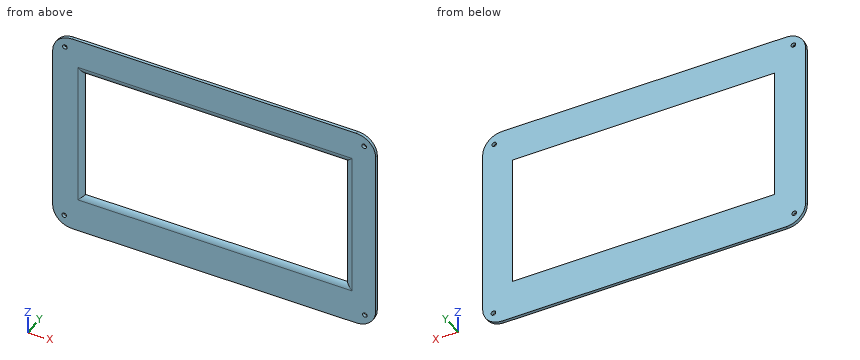
from build123d import *

# Parameters (mm, degrees)
F0_W         = 170.18
F0_H         = 87.63
F1_DEPTH     = 2
F3_D         = 3
F4_T1_DEPTH  = 87.63
F4_T3_DEPTH  = 170.18
F4_T9_DEPTH  = 97.7295049384
F4_T13_DEPTH = 180.2795049384
F4_T20_DEPTH = 97.7295049384
F4_T24_DEPTH = 180.2795049384
F4_T31_DEPTH = 180.2795049384
F4_T35_DEPTH = 97.7295049384
F4_T42_DEPTH = 180.2795049384
F4_T46_DEPTH = 97.7295049384


# Not quite as in the source:
# - a fillet or chamfer that OpenCascade refuses, or shapes differently, is made with other operations: its cross-section is extruded or revolved along the edge and cut away or added


with BuildPart() as f1:
    # F0 (on Front) → F1 (new body)
    with BuildSketch(Plane.XZ):
        with BuildLine():
            Line((94.3139557123, 80.8203592896), (-90.2860442877, 80.8203592896))
            ThreePointArc((-90.2860442877, 80.8203592896), (-99.2663004088, 77.1006154107), (-102.9860442877, 68.1203592896))
            Line((-102.9860442877, 68.1203592896), (-102.9860442877, -43.4872407104))
            ThreePointArc((-102.9860442877, -43.4872407104), (-99.2663004088, -52.4674968314), (-90.2860442877, -56.1872407104))
            Line((-90.2860442877, -56.1872407104), (94.3139557123, -56.1872407104))
            ThreePointArc((94.3139557123, -56.1872407104), (103.2942118334, -52.4674968314), (107.0139557123, -43.4872407104))
            Line((107.0139557123, -43.4872407104), (107.0139557123, 68.1203592896))
            ThreePointArc((107.0139557123, 68.1203592896), (103.2942118334, 77.1006154107), (94.3139557123, 80.8203592896))
        make_face()
        with Locations((2.4907932702, 13.8051814874)):
            Rectangle(F0_W, F0_H, mode=Mode.SUBTRACT)
    extrude(amount=F1_DEPTH)

    # F3 (through all)
    with Locations(Plane.XZ.offset(2)):
        with Locations((-95.5433249474, -48.3972094953), (-95.0444117188, 73.3367204666), (100.0292077661, -48.3972094953), (99.5303019881, 73.3367204666)):
            Hole(F3_D / 2)

    # F4: fillet of radius 5.08 on 4 edges, made by hand

    # F4_s2 → F4_t1 (cut)
    with BuildSketch(Plane.XY.offset(-30.0098185126)):
        with BuildLine():
            ThreePointArc((91.6205952456, -2), (89.3667097117, -1.4726256161), (87.5807932702, 0))
            Line((87.5807932702, 0), (87.5807932702, -2))
            Line((87.5807932702, -2), (91.6205952456, -2))
        make_face()
        with BuildLine():
            ThreePointArc((-86.6390087051, -2), (-84.3851231712, -1.4726256161), (-82.5992067298, 0))
            Line((-82.5992067298, 0), (-82.5992067298, -2))
            Line((-82.5992067298, -2), (-86.6390087051, -2))
        make_face()
    extrude(amount=F4_T1_DEPTH, mode=Mode.SUBTRACT)

    # F4_s4 → F4_t3 (cut)
    with BuildSketch(Plane.YZ.offset(-82.5992067298)):
        with BuildLine():
            ThreePointArc((-2, 61.6599834627), (-1.4726256161, 59.4060979288), (0, 57.6201814874))
            Line((0, 57.6201814874), (-2, 57.6201814874))
            Line((-2, 57.6201814874), (-2, 61.6599834627))
        make_face()
        with BuildLine():
            ThreePointArc((-2, -34.049620488), (-1.4726256161, -31.795734954), (0, -30.0098185126))
            Line((0, -30.0098185126), (-2, -30.0098185126))
            Line((-2, -30.0098185126), (-2, -34.049620488))
        make_face()
    extrude(amount=F4_T3_DEPTH, mode=Mode.SUBTRACT)


with BuildPart() as f4_tool7:
    # F4_s8 → F4_t9 (new body)
    with BuildSketch(Plane.XY.offset(67.7196864257)):
        with BuildLine():
            ThreePointArc((91.6205952456, -2), (89.3667097117, -1.4726256161), (87.5807932702, 0))
            Line((87.5807932702, 0), (87.5807932702, -2))
            Line((87.5807932702, -2), (91.6205952456, -2))
        make_face()
    extrude(amount=-F4_T9_DEPTH)

    split(bisect_by=Plane.XY.offset(57.6201814874), keep=Keep.TOP)


with BuildPart() as f4_tool11:
    # F4_s12 → F4_t13 (new body)
    with BuildSketch(Plane.YZ.offset(-82.5992067298)):
        with BuildLine():
            ThreePointArc((-2, 61.6599834627), (-1.4726256161, 59.4060979288), (0, 57.6201814874))
            Line((0, 57.6201814874), (-2, 57.6201814874))
            Line((-2, 57.6201814874), (-2, 61.6599834627))
        make_face()
    extrude(amount=F4_T13_DEPTH)

    split(bisect_by=Plane.YZ.offset(87.5807932702), keep=Keep.TOP)


with BuildPart() as f4_tool7_1:
    add(f4_tool7.part)

    # F4_t15: intersect F4_tool11
    add(f4_tool11.part, mode=Mode.INTERSECT)


with BuildPart() as f1_1:
    add(f1.part)

    # F4_t5: cut F4_tool7
    add(f4_tool7_1.part, mode=Mode.SUBTRACT)


with BuildPart() as f4_tool18:
    # F4_s19 → F4_t20 (new body)
    with BuildSketch(Plane.XY.offset(57.6201814874)):
        with BuildLine():
            ThreePointArc((91.6205952456, -2), (89.3667097117, -1.4726256161), (87.5807932702, 0))
            Line((87.5807932702, 0), (87.5807932702, -2))
            Line((87.5807932702, -2), (91.6205952456, -2))
        make_face()
    extrude(amount=-F4_T20_DEPTH)

    split(bisect_by=Plane.XY.offset(-30.0098185126), keep=Keep.BOTTOM)


with BuildPart() as f4_tool22:
    # F4_s23 → F4_t24 (new body)
    with BuildSketch(Plane.YZ.offset(97.6802982086)):
        with BuildLine():
            ThreePointArc((-2, -34.049620488), (-1.4726256161, -31.795734954), (0, -30.0098185126))
            Line((0, -30.0098185126), (-2, -30.0098185126))
            Line((-2, -30.0098185126), (-2, -34.049620488))
        make_face()
    extrude(amount=-F4_T24_DEPTH)

    split(bisect_by=Plane.YZ.offset(87.5807932702), keep=Keep.TOP)


with BuildPart() as f4_tool18_1:
    add(f4_tool18.part)

    # F4_t26: intersect F4_tool22
    add(f4_tool22.part, mode=Mode.INTERSECT)


with BuildPart() as f1_2:
    add(f1_1.part)

    # F4_t16: cut F4_tool18
    add(f4_tool18_1.part, mode=Mode.SUBTRACT)


with BuildPart() as f4_tool29:
    # F4_s30 → F4_t31 (new body)
    with BuildSketch(Plane.YZ.offset(-92.6987116681)):
        with BuildLine():
            ThreePointArc((-2, 61.6599834627), (-1.4726256161, 59.4060979288), (0, 57.6201814874))
            Line((0, 57.6201814874), (-2, 57.6201814874))
            Line((-2, 57.6201814874), (-2, 61.6599834627))
        make_face()
    extrude(amount=F4_T31_DEPTH)

    split(bisect_by=Plane.YZ.offset(-82.5992067298), keep=Keep.BOTTOM)


with BuildPart() as f4_tool33:
    # F4_s34 → F4_t35 (new body)
    with BuildSketch(Plane.XY.offset(-30.0098185126)):
        with BuildLine():
            ThreePointArc((-86.6390087051, -2), (-84.3851231712, -1.4726256161), (-82.5992067298, 0))
            Line((-82.5992067298, 0), (-82.5992067298, -2))
            Line((-82.5992067298, -2), (-86.6390087051, -2))
        make_face()
    extrude(amount=F4_T35_DEPTH)

    split(bisect_by=Plane.XY.offset(57.6201814874), keep=Keep.TOP)


with BuildPart() as f4_tool29_1:
    add(f4_tool29.part)

    # F4_t37: intersect F4_tool33
    add(f4_tool33.part, mode=Mode.INTERSECT)


with BuildPart() as f1_3:
    add(f1_2.part)

    # F4_t27: cut F4_tool29
    add(f4_tool29_1.part, mode=Mode.SUBTRACT)


with BuildPart() as f4_tool40:
    # F4_s41 → F4_t42 (new body)
    with BuildSketch(Plane.YZ.offset(87.5807932702)):
        with BuildLine():
            ThreePointArc((-2, -34.049620488), (-1.4726256161, -31.795734954), (0, -30.0098185126))
            Line((0, -30.0098185126), (-2, -30.0098185126))
            Line((-2, -30.0098185126), (-2, -34.049620488))
        make_face()
    extrude(amount=-F4_T42_DEPTH)

    split(bisect_by=Plane.YZ.offset(-82.5992067298), keep=Keep.BOTTOM)


with BuildPart() as f4_tool44:
    # F4_s45 → F4_t46 (new body)
    with BuildSketch(Plane.XY.offset(-40.109323451)):
        with BuildLine():
            ThreePointArc((-86.6390087051, -2), (-84.3851231712, -1.4726256161), (-82.5992067298, 0))
            Line((-82.5992067298, 0), (-82.5992067298, -2))
            Line((-82.5992067298, -2), (-86.6390087051, -2))
        make_face()
    extrude(amount=F4_T46_DEPTH)

    split(bisect_by=Plane.XY.offset(-30.0098185126), keep=Keep.BOTTOM)


with BuildPart() as f4_tool40_1:
    add(f4_tool40.part)

    # F4_t48: intersect F4_tool44
    add(f4_tool44.part, mode=Mode.INTERSECT)


with BuildPart() as f1_4:
    add(f1_3.part)

    # F4_t38: cut F4_tool40
    add(f4_tool40_1.part, mode=Mode.SUBTRACT)


solid = f1_4.part
Build history of the part. All positions in model axes, mm. Coordinates: 2 decimals unless noted, no trailing zeros. Order: outer loops, then holes, each group sorted by start corner. A loop starts at its lowest first (then second) coordinate and runs counter-clockwise, first axis right, second up. Notation, with made-up numbers: (74, 58.5) - (92, 58.5) arc R26 ccw to (92, 93.5) - close; hole circle Ø1 at (64, 32). An arc over 180 degrees is marked (long way). Put each result on its own line as item: value.
1. Saw through at B-B (x = 19). Write the cut outline in (y, z), and give its area (3 significant figures).
Answer sheet:
outline: (-2, -56.19) - (0, -56.19) - (0, -30.01) arc R5.08 ccw to (-2, -34.05) - close; (-2, 61.66) arc R5.08 ccw to (0, 57.62) - (0, 80.82) - (-2, 80.82) - close
area: 93.9 mm^2
2. Saw through at A-A (z = 10). Write the cut outline in (x, y).
Answer sheet:
outline: (-102.99, -2) - (-86.64, -2) arc R5.08 ccw to (-82.6, 0) - (-102.99, 0) - close; (87.58, 0) arc R5.08 ccw to (91.62, -2) - (107.01, -2) - (107.01, 0) - close
3. Drop a flat-ended pin along its axis: P1, Ø2.5, axis at x = 100.03, z = -48.4, coming from the +Y side. Give the stop position or say it passes through.
Answer sheet:
P1: passes through
4. Saw through at C-C (y = -0.6). Write the cut outline in (x, z), and give its area (3 significant figures).
Answer sheet:
outline: (-102.99, -43.49) arc R12.7 ccw to (-90.29, -56.19) - (94.31, -56.19) arc R12.7 ccw to (107.01, -43.49) - (107.01, 68.12) arc R12.7 ccw to (94.31, 80.82) - (-90.29, 80.82) arc R12.7 ccw to (-102.99, 68.12) - close; hole circle Ø3 at (-95.54, -48.4); hole circle Ø3 at (-95.04, 73.34); hole (-83.14, -30.55) - (88.12, -30.55) - (88.12, 58.16) - (-83.14, 58.16) - close; hole circle Ø3 at (99.53, 73.34); hole circle Ø3 at (100.03, -48.4)
area: 13,400 mm^2
5. Probe line 1 along Y through (x, z) = (-86.5, -32); line 2 along X through (y, z) = (-0.65, -5); line 3 along X through (y, z) = (-1, 11). List the from-to ranges inside material, lowest first. Write a range as [from, to].
Answer sheet:
line 1: y = [-2, 0]
line 2: x = [-102.99, -83.19], [88.17, 107.01]
line 3: x = [-102.99, -83.61], [88.59, 107.01]
